Check sheet for the modelled part. Datum: model origin and axes. Units: mm. A direction names the side the tool comes from. Give positions to 0.01 mm unless a question says otherwise; leave off trailing zeros. Order: outer loops, then holes, each group sorted by start corner. A loop starts at its lowest first (then second) coordinate and runs counter-clockwise, first axis right, second up. Notation, with made-up numbers: (14.25, 49.5) -> (51.25, 49.5) arc R27 cw to (51.25, 88.5) -> close; hole circle Ø2 at (64, 81.5). An arc over 180 degrees is marked (long way). Answer in a Markdown table with one row per item. Add a question column.
(1) Release check for a two-part mould opening along X. For faces 5 (the face through (28.89, 52.94, 2.46)), 6 (the face through (-32.5, 44, 2)), 7 (the face through (18, 90, 2)) record: released by +X, released by -X, zero draft, split by the parting line, or undercut.
(2) Cross-section at A-A (y = 57.5). Record the cut outline in (x, z).
(3) Cross-section at D-D (x = -28). Record the cut outline in (y, z), then the cut area to 3 significant figures.
(4) Go/stop test with flat-tipped pins: pin 1 (2 mm diameter, centred on x = -27.5, y = 62.5, fed in from -Z); pin 2 (2 mm diameter, centred on x = 8.5, z = 1.5, fed in from -Y); pin 3 (1.6 mm diameter, centred on x = 11.5, z = 4.5, fed in from -Y); pin 4 (1.6 mm diameter, centred on x = 12.5, z = 4, fed in from -Y). Record where each tip stops, or that it passes through.
(5) Cross-section at B-B (x = 19.5). Record the cut outline in (y, z).
(6) Set-up check for faces 1 (the face through (-4.504, 84, 3)), 2 (the face through (-13, 78, 3)), 3 (the face through (0, 30, 0)), 4 (the face through (-10.6, 13.3, 3)): record each of +Z, -Z, +X, -X, +Y, -Y from which the full face is reachable in a straight line by a thin tool's end or side.
(7) Thickness scan on L1, parallel to X at y = 12, z = 4.4; L2, parallel to Y at x = 0, z = 0.5; L3, parallel to X at y = 57, z = 3. Record the ranges inside material, lowest first. Write a range as [from, to].
(8) Cross-section at C-C (z = 2.05). State how many separate pieces and enclosed holes the cut face has, then the cut area to 3 significant figures.
```python
from build123d import *

# Parameters (mm, degrees)
BOSS_EXTRUDE1_DEPTH = 5
SKETCH2_R           = 6
CUT_EXTRUDE1_DEPTH  = 96.818839484
SKETCH3_R           = 8
CUT_EXTRUDE2_DEPTH  = 4
SKETCH4_R           = 1.75
CUT_EXTRUDE3_DEPTH  = 96.818839484
CUT_EXTRUDE4_DEPTH  = 96.818839484
CUT_EXTRUDE6_DEPTH  = 2
SKETCH8_R           = 1.75
CUT_EXTRUDE7_DEPTH  = 96.818839484


with BuildPart() as part:
    # Sketch1 → Boss-Extrude1 (new body)
    with BuildSketch(Plane.XY):
        with BuildLine():
            Line((-32.5, 0), (-32.5, 90))
            Line((-32.5, 90), (32.5, 90))
            Line((32.5, 90), (32.5, 0))
            ThreePointArc((32.5, 0), (0, -32.5), (-32.5, 0))
        make_face()
    extrude(amount=BOSS_EXTRUDE1_DEPTH)

    # Sketch2 → Cut-Extrude1 (cut, through all)
    with BuildSketch(Plane.XY.offset(5)):
        Circle(SKETCH2_R)
    extrude(amount=-CUT_EXTRUDE1_DEPTH, mode=Mode.SUBTRACT)

    # Sketch3 → Cut-Extrude2 (cut)
    with BuildSketch(Plane.XY.offset(5)):
        Circle(SKETCH3_R)
    extrude(amount=-CUT_EXTRUDE2_DEPTH, mode=Mode.SUBTRACT)

    # Sketch4 → Cut-Extrude3 (cut, through all)
    with BuildSketch(Plane.XY.offset(5)):
        with Locations((-12, 12)):
            Circle(SKETCH4_R)
        with Locations(Location((12, 12, 0), (0, 0, 180))):
            Circle(SKETCH4_R)
        with Locations((12, -12)):
            Circle(SKETCH4_R)
        with Locations(Location((-12, -12, 0), (0, 0, 180))):
            Circle(SKETCH4_R)
    extrude(amount=-CUT_EXTRUDE3_DEPTH, mode=Mode.SUBTRACT)

    # Sketch5 → Cut-Extrude4 (cut, through all)
    with BuildSketch(Plane.XY.offset(5)):
        Polygon((-21.5, 78), (-4.504076159, 78), (-4.504076159, 90), (4.504076159, 90), (4.504076159, 78), (21.5, 78), (21.5, 39), (-21.5, 39), align=None)
    extrude(amount=-CUT_EXTRUDE4_DEPTH, mode=Mode.SUBTRACT)

    # Sketch7 → Cut-Extrude6 (cut)
    with BuildSketch(Plane.XY.offset(5)):
        Polygon((-8.709103466, 12), (-10.354551733, 14.85), (-13.645448267, 14.85), (-15.290896534, 12), (-13.645448267, 9.15), (-10.354551733, 9.15), align=None)
        Polygon((10.354551733, 9.15), (8.709103466, 12), (10.354551733, 14.85), (13.645448267, 14.85), (15.290896534, 12), (13.645448267, 9.15), align=None)
        Polygon((8.709103466, -12), (10.354551733, -14.85), (13.645448267, -14.85), (15.290896534, -12), (13.645448267, -9.15), (10.354551733, -9.15), align=None)
        Polygon((-10.354551733, -9.15), (-8.709103466, -12), (-10.354551733, -14.85), (-13.645448267, -14.85), (-15.290896534, -12), (-13.645448267, -9.15), align=None)
    extrude(amount=-CUT_EXTRUDE6_DEPTH, mode=Mode.SUBTRACT)

    # Sketch8 → Cut-Extrude7 (cut, through all)
    with BuildSketch(Plane(origin=(0, 0, 0), x_dir=(-1, 0, 0), z_dir=(0, 0, -1))):
        with Locations((-27.5, 62.5)):
            Circle(SKETCH8_R)
        with Locations((-27.5, 54)):
            Circle(SKETCH8_R)
        with Locations(Location((27.5, 54, 0), (0, 0, 180))):
            Circle(SKETCH8_R)
        with Locations(Location((27.5, 62.5, 0), (0, 0, 180))):
            Circle(SKETCH8_R)
    extrude(amount=-CUT_EXTRUDE7_DEPTH, mode=Mode.SUBTRACT)


solid = part.part
```
Answer below:
| question | item | result |
|---|---|---|
| 1 | face 5 | undercut |
| 1 | face 6 | released by -X |
| 1 | face 7 | zero draft |
| 2 | outline | (-32.5, 0) -> (-21.5, 0) -> (-21.5, 5) -> (-32.5, 5) -> close; (21.5, 0) -> (32.5, 0) -> (32.5, 5) -> (21.5, 5) -> close |
| 3 | outline | (-16.5, 0) -> (52.32, 0) -> (52.32, 5) -> (-16.5, 5) -> close; (55.68, 0) -> (60.82, 0) -> (60.82, 5) -> (55.68, 5) -> close; (64.18, 0) -> (90, 0) -> (90, 5) -> (64.18, 5) -> close |
| 3 | area | 499 mm² |
| 4 | pin 1 | passes through |
| 4 | pin 2 | stops at y = -31.62 |
| 4 | pin 3 | stops at y = -30.69 |
| 4 | pin 4 | stops at y = -30.32 |
| 5 | outline | (-26, 0) -> (39, 0) -> (39, 5) -> (-26, 5) -> close; (78, 0) -> (90, 0) -> (90, 5) -> (78, 5) -> close |
| 6 | face 1 | +Z, -Z, +Y |
| 6 | face 2 | +Z, -Z |
| 6 | face 3 | -Z, +X, -X, +Y, -Y |
| 6 | face 4 | +Z |
| 7 | L1 | x = [-32.5, -15.29], [-8.71, 8.71], [15.29, 32.5] |
| 7 | L2 | y = [-32.5, -6], [6, 39] |
| 7 | L3 | x = [-32.5, -21.5], [21.5, 32.5] |
| 8 | separate pieces | 1 |
| 8 | enclosed holes | 9 |
| 8 | area | 5,450 mm² |
